The drawing under review shows one solid part. Ordinate dimensions are in mm from its lowest x, y, z. Give positions to 0.01 mm unless a question says otherwise; leave off trailing zeros. Write each loop counter-clockwise with the first axis right and the second up, starting at its lowest first coordinate (ties: lowest second). Pieces come first, ordered by that corner, then holes.
Q1. We need section A-A (x = 124.5). Write out the cut boundary in (y, z) (1 decimal).
Q2. We need section B-B (y = 108.5). Write out the cut boundary in (x, z) (1 decimal).
Q3. We need section D-D (y = 14). Write out the cut boundary in (x, z).
Q4. Mouldability with a two-part tool opening along Y and no side actions: class the marked faces 1, 2 and 3 as released by +Y, released by -Y, zero draft, split by the parting line, or undercut.
Q5. For line 1 (Y direction, x = 72.5, z = 131); line 2 (Y direction, x = 88, z = 82) (1 decimal); line 3 (X direction, y = 90.5, z = 28) (1 decimal), list the stretches that pass through material, from the lowest coordinate up.
Q6. We need section C-C (z = 182.5). Write out the cut boundary in (x, y) (1 decimal), then the cut area to 3 significant figures.
Q7. Insertion check: P1, Ø12, axis at x = 86.5, z = 121.5, coming from the -Y side; P2, Ø5, axis at y = 74, z = 152.5, coming from the -X side; P3, Ø2, axis at y = 119, z = 98.5, coming from the +X side; P4, Ø1.5, axis at x = 38, z = 166, coming from the +Y side. Each pin has a flat end and moves straight along its axis. Give the tip position at first contact, or say it passes through.
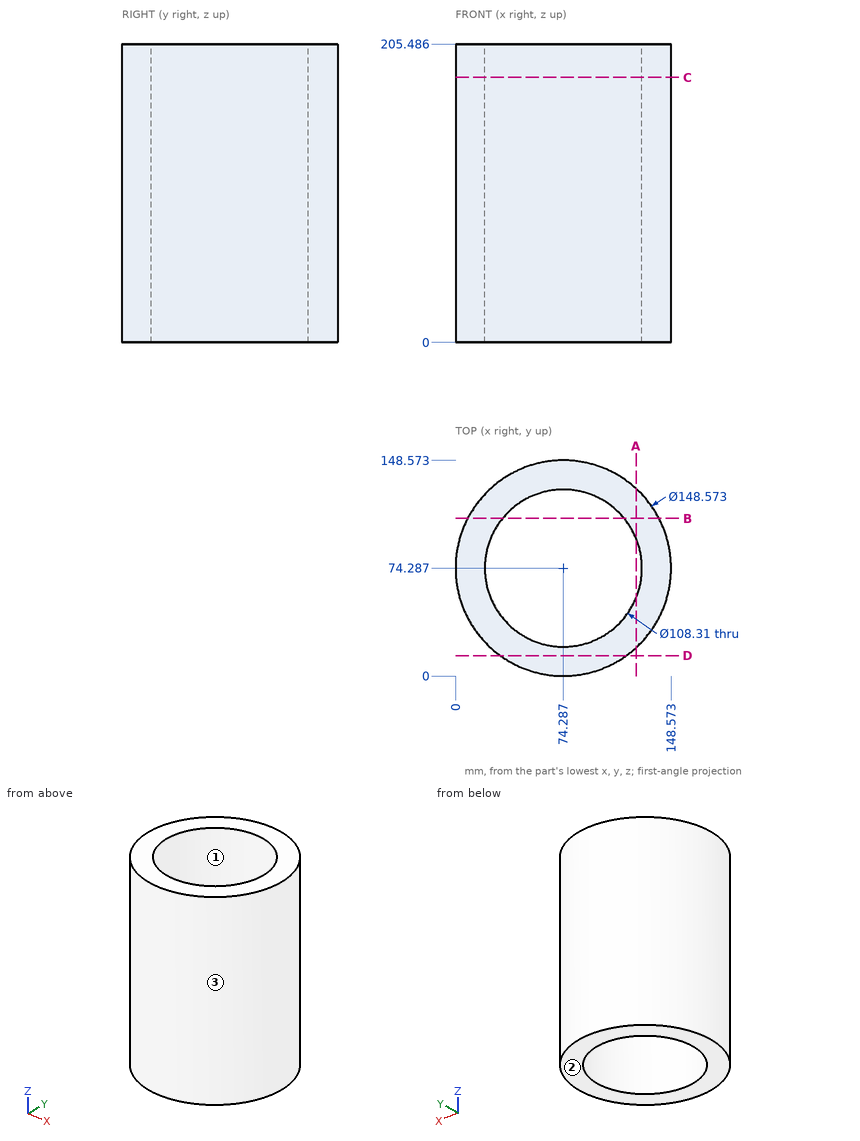
Computed:
1. outline: (19.5, 0) - (54, 0) - (54, 205.5) - (19.5, 205.5) - close; (94.6, 0) - (129, 0) - (129, 205.5) - (94.6, 205.5) - close
2. outline: (8.3, 0) - (32.3, 0) - (32.3, 205.5) - (8.3, 205.5) - close; (116.3, 0) - (140.2, 0) - (140.2, 205.5) - (116.3, 205.5) - close
3. outline: (30.88, 0) - (117.69, 0) - (117.69, 205.49) - (30.88, 205.49) - close
4. face 1: undercut
4. face 2: zero draft
4. face 3: split by the parting line
5. line 1: y = 0.02 to 20.16, 128.41 to 148.55
5. line 2: y = 1.3 to 21.9, 126.7 to 147.3
5. line 3: x = 1.8 to 22.6, 126 to 146.8
6. outline: circle Ø148.6 at (74.3, 74.3); hole circle Ø108.3 at (74.3, 74.3)
6. area: 8,120 mm2
7. P1: stops at y = 0.26
7. P2: stops at x = 0
7. P3: stops at x = 134.35
7. P4: stops at y = 139.52
